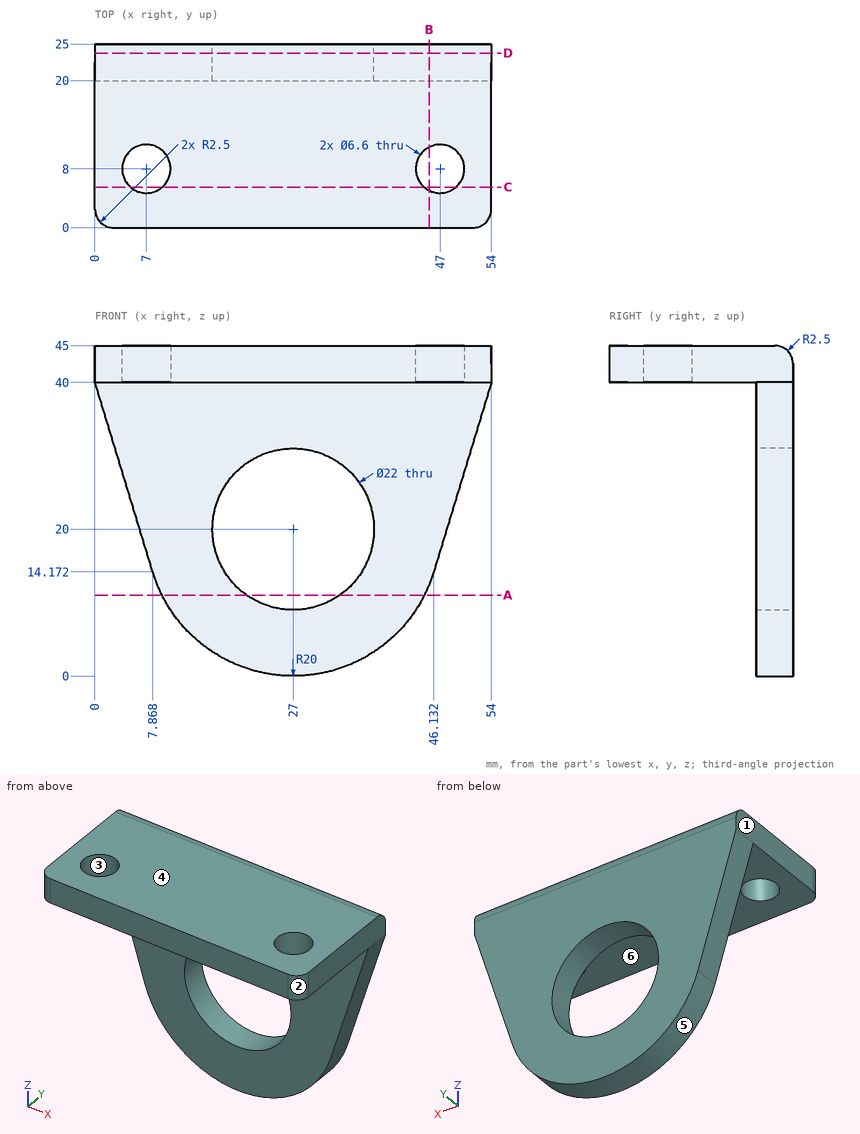
Geometry check sheet. Reference: drawing and pictorial views, mm from the part's lowest x, y, z. A direction names the side the tool comes from. Give positions to 0.01 mm unless a question says otherwise; leave off trailing zeros. Order: outer loops, then holes, each group sorted by start corner. A loop starts at its lowest first (then second) coordinate and runs counter-clockwise, first axis right, second up. Notation, with made-up numbers: (-35, 9) - (-21, 9) arc R6 cw to (-21, 15) - close; hole circle Ø3 at (-1, -20.75). An arc over 180 degrees is marked (long way). Use one line per item in the form item = value.
1) Draft check along X on the marked faces 1, 2, 3 and 4. Enter one of: released by +X, released by -X, zero draft, split by the parting line, or undercut.
Working result:
face_1 = released by -X
face_2 = released by +X
face_3 = undercut
face_4 = zero draft
2) Sectioned sample at B-B (x = 45.5). Record the boundary of the cut face in (y, z).
Working result:
outline = (0, 40) - (5.06, 40) - (5.06, 45) - (0, 45) - close; (10.94, 40) - (20, 40) - (20, 12.4) - (25, 12.4) - (25, 42.5) arc R2.5 ccw to (22.5, 45) - (10.94, 45) - close
3) Material ranges on probe 1 along Y at (x, z) = (16.5, 15); probe 2 along Y at (x, z) = (47, 42); probe 3 along Z at (x, y) = (2.5, 4), recorded low to high. Write a range as from..to.
Working result:
probe_1 = 20..25
probe_2 = 0..4.7, 11.3..25
probe_3 = 40..45
4) Depth check by flat-ended pin: pin 1 Ø10 at (x, z) = (28.5, 27.5) entering from +Y; pin 2 Ø1.5 at (y, z) = (22.5, 9.5) entering from -X; pin 3 Ø5 at (x, z) = (45.5, 10.5) entering from -Y. Enter the tip coordinate at first touch or a pass-through.
Working result:
pin_1 = 25
pin_2 = 9.54
pin_3 = 20
5) Sectioned sample at C-C (y = 5.5). Record the boundary of the cut face in (x, z), and give its area (3 significant figures).
Working result:
outline = (0, 40) - (4.85, 40) - (4.85, 45) - (0, 45) - close; (9.15, 40) - (44.85, 40) - (44.85, 45) - (9.15, 45) - close; (49.15, 40) - (54, 40) - (54, 45) - (49.15, 45) - close
area = 227 mm^2
6) Sectioned sample at A-A (z = 11). Record the boundary of the cut face in (x, y).
Working result:
outline = (9.14, 20) - (20.68, 20) - (20.68, 25) - (9.14, 25) - close; (33.32, 20) - (44.86, 20) - (44.86, 25) - (33.32, 25) - close
7) Sectioned sample at D-D (y = 23.75). Record the boundary of the cut face in (x, z) (1 decimal).
Working result:
outline = (0, 40) - (7.9, 14.2) arc R20 ccw to (46.1, 14.2) - (54, 40) - (54, 44.7) - (0, 44.7) - close; hole circle Ø22 at (27, 20)
8) Access from +Z, -Z, +X, -X, +Y, -Y to the whole of each face (thin tool, end or side, straight path). Record for the marked faces 5 and 6.
Working result:
face_5 = -Z, +Y, -Y
face_6 = -Z, +X, -X, -Y
